from build123d import *

# Parameters (mm, degrees)
SKIZZE1_W                       = 100
SKIZZE1_H                       = 100
AUFSATZ_LINEAR_AUSTRAGEN1_DEPTH = 50
SKIZZE5_W                       = 10
SKIZZE5_H                       = 20


with BuildPart() as part:
    # Skizze1 → Aufsatz-Linear austragen1 (new body)
    with BuildSketch(Plane.XY):
        Rectangle(SKIZZE1_W, SKIZZE1_H)
    extrude(amount=AUFSATZ_LINEAR_AUSTRAGEN1_DEPTH)

    # Schnitt-Austragung1: sweep along a path in Skizze2
    with BuildLine(Plane.XY.offset(50)) as schnitt_austragung1_path:
        CenterArc((0, 0), 25, 0, 360)
    # Skizze5 → Schnitt-Austragung1 (sweep, cut)
    with BuildSketch(Plane(origin=(0, 0, 0), x_dir=(1, 0, 0), z_dir=(0, 1, 0))):
        with Locations((-25, -50)):
            Rectangle(SKIZZE5_W, SKIZZE5_H)
    sweep(path=schnitt_austragung1_path.line, mode=Mode.SUBTRACT)


solid = part.part
Verification items for the finished model (mm, model axes). Coordinates: 2 decimals unless noted, no trailing zeros. Loops run counter-clockwise (first coordinate to the right, second up) from the corner with the lowest first, then second, coordinate; pieces in that order, holes last. Notation, with made-up numbers: (5.25, -31.75) -> (24.25, -31.75) arc R20 ccw to (24.25, -5.75) -> close; hole circle Ø4 at (75, -19.5). An arc over 180 degrees is marked (long way). Answer as a JSON object with one key per item and string values. Group by question number.
Item 1: Sectioned sample at A-A on z = 43. Record the boundary of the cut face in (x, y), plus the area to 3 significant figures.
Item 2: Scan lines: probe 1 along Y at (x, z) = (0, 45); probe 2 along Y at (x, z) = (-7, 44) (3 decimals); probe 3 along X at (y, z) = (-3, 46). Record each from-to range of solid material in increasing order.
Item 3: Depth check by flat-ended pin: pin 1 (10 mm diameter, centred on x = 38.5, y = 33.5, fed in from -Z). Enter the tip coordinate at first touch or a pass-through.
Item 4: Mould release check, pull along X, two halves, no side actions. Record for faces 1 (the cylindrical face through (19.076, 6.007, 44.93)), 2 (the flat face through (50, -1, 25)), 3 (the flat face through (0, 0, 50)), 4 (the cylindrical face through (-6.503, -29.287, 45.07)): +X half, -X half, draft (parallel to the pull), parting line (faces both ways), or undercut.
Evaluation:
{
 "1": {"outline": "(-50, -50) -> (50, -50) -> (50, 50) -> (-50, 50) -> close; circle Ø40 at (0, 0); hole circle Ø60 at (0, 0)", "area": "8,430 mm²"},
 "2": {"probe 1": "y = -50 to -30, -20 to 20, 30 to 50", "probe 2": "y = -50 to -29.172, -18.735 to 18.735, 29.172 to 50", "probe 3": "x = -50 to -29.85, -19.77 to 19.77, 29.85 to 50"},
 "3": {"pin 1": "stops at z = 0"},
 "4": {"face 1": "undercut", "face 2": "+X half", "face 3": "draft", "face 4": "undercut"}
}
